```python
from build123d import *

# Parameters (mm, degrees)
F0_R          = 1.75
F1_DEPTH      = 15.875
F3_DEPTH      = 31.75
F4_R          = 3
F5_W          = 5
F5_H          = 35
F6_DEPTH      = 10.001
F6_DEPTH_BACK = 7.5573491861
F7_T1_DEPTH   = 8.7055800262
F7_T3_DEPTH   = 8.75
F7_T5_DEPTH   = 8.75
F7_T7_DEPTH   = 8.7055800262
F8_DEPTH      = 0.2
F9_DEPTH      = 0.2


# Not quite as in the source:
# - a fillet or chamfer that OpenCascade refuses, or shapes differently, is made with other operations: its cross-section is extruded or revolved along the edge and cut away or added


with BuildPart() as f1:
    # F0 (on Right) → F1 (new body, symmetric)
    with BuildSketch(Plane.YZ):
        with BuildLine():
            Line((-5.2303039929, -1.5), (-4.7696960071, -1.5))
            ThreePointArc((-4.7696960071, -1.5), (5, 0), (-4.7696960071, 1.5))
            Line((-4.7696960071, 1.5), (-35, 1.5))
            Line((-35, 1.5), (-42.5, -6))
            Line((-42.5, -6), (-77.5, -6))
            Line((-77.5, -6), (-90.4705627485, 6.9705627485))
            ThreePointArc((-90.4705627485, 6.9705627485), (-93.2989898732, 6.9705627485), (-93.2989898732, 4.1421356237))
            Line((-93.2989898732, 4.1421356237), (-79.1568542495, -10))
            Line((-79.1568542495, -10), (-40.8431457505, -10))
            Line((-40.8431457505, -10), (-32.3431457505, -1.5))
            Line((-32.3431457505, -1.5), (-14.7696960071, -1.5))
            ThreePointArc((-14.7696960071, -1.5), (-10, -5), (-5.2303039929, -1.5))
        make_face()
        Circle(F0_R, mode=Mode.SUBTRACT)
    extrude(amount=F1_DEPTH, both=True)

    # F2 (on face) → F3 (join, through all)
    with BuildSketch(Plane.YZ.offset(15.875)):
        with BuildLine():
            ThreePointArc((-5.2303039929, -1.5), (-7.0419601085, -4.0311288741), (-10, -5))
            Line((-10, -5), (0, -5))
            ThreePointArc((0, -5), (-2.9580398915, -4.0311288741), (-4.7696960071, -1.5))
            Line((-4.7696960071, -1.5), (-5.2303039929, -1.5))
        make_face()
    extrude(amount=-F3_DEPTH)

    # F4
    f4_edges = [f1.edges().sort_by_distance(p)[0] for p in [
        (0, -4.769696, 1.5),
        (0, -14.769696, -1.5),
        (0, -77.5, -6),
        (0, -79.156854, -10),
        (0, -40.843146, -10),
        (0, -32.343146, -1.5),
        (0, -42.5, -6),
        (0, -35, 1.5),
    ]]
    fillet(f4_edges, radius=F4_R)

    # F5 (on Top) → F6 (cut, two sides)
    with BuildSketch(Plane.XY) as f6_sk:
        with Locations((-13.375, -12.5)):
            Rectangle(F5_W, F5_H)
        with Locations((13.375, -12.5)):
            Rectangle(F5_W, F5_H)
    extrude(amount=-F6_DEPTH, mode=Mode.SUBTRACT)
    extrude(f6_sk.sketch, amount=F6_DEPTH_BACK, mode=Mode.SUBTRACT)

    # F7: fillet of radius 1.5 on 4 edges, made by hand

    # F7_s2 → F7_t1 (cut)
    with BuildSketch(Plane.YZ.offset(10.875)):
        with BuildLine():
            ThreePointArc((-31.3668350211, -1.5118453264), (-30.3932598615, -1.0302531824), (-30, -0.0177679895))
            Line((-30, -0.0177679895), (-29.85, -0.0177679895))
            Line((-29.85, -0.0177679895), (-29.85, -1.5))
            Line((-29.85, -1.5), (-30, -1.65))
            ThreePointArc((-30, -1.65), (-31.1005050634, -1.65), (-31.3535185232, -1.66125306))
            Line((-31.3535185232, -1.66125306), (-31.3668350211, -1.5118453264))
        make_face()
    extrude(amount=F7_T1_DEPTH, mode=Mode.SUBTRACT)

    # F7_s4 → F7_t3 (cut)
    with BuildSketch(Plane.YZ.offset(10.875)):
        with BuildLine():
            ThreePointArc((-30, 0), (-30.4393398282, 1.0606601718), (-31.5, 1.5))
            Line((-31.5, 1.5), (-30, 1.5))
            Line((-30, 1.5), (-30, 0))
        make_face()
    extrude(amount=F7_T3_DEPTH, mode=Mode.SUBTRACT)

    # F7_s6 → F7_t5 (cut)
    with BuildSketch(Plane.YZ.offset(-19.625)):
        with BuildLine():
            ThreePointArc((-30, 0), (-30.4393398282, 1.0606601718), (-31.5, 1.5))
            Line((-31.5, 1.5), (-30, 1.5))
            Line((-30, 1.5), (-30, 0))
        make_face()
    extrude(amount=F7_T5_DEPTH, mode=Mode.SUBTRACT)

    # F7_s8 → F7_t7 (cut)
    with BuildSketch(Plane.YZ.offset(-19.5805800262)):
        with BuildLine():
            ThreePointArc((-31.3668350211, -1.5118453264), (-30.3932598615, -1.0302531824), (-30, -0.0177679895))
            Line((-30, -0.0177679895), (-29.85, -0.0177679895))
            Line((-29.85, -0.0177679895), (-29.85, -1.5))
            Line((-29.85, -1.5), (-30, -1.65))
            ThreePointArc((-30, -1.65), (-31.1005050634, -1.65), (-31.3535185232, -1.66125306))
            Line((-31.3535185232, -1.66125306), (-31.3668350211, -1.5118453264))
        make_face()
    extrude(amount=F7_T7_DEPTH, mode=Mode.SUBTRACT)

    # F8 (cut): a face of the model
    f8_faces = [f1.faces().sort_by_distance(p)[0] for p in [
        (10.875, -9.1101781633, -0.6280033564),
    ]]
    extrude(f8_faces, amount=-F8_DEPTH, mode=Mode.SUBTRACT)

    # F9 (cut): a face of the model
    f9_faces = [f1.faces().sort_by_distance(p)[0] for p in [
        (-10.875, -9.1101781633, -0.6280033564),
    ]]
    extrude(f9_faces, amount=-F9_DEPTH, mode=Mode.SUBTRACT)


solid = f1.part
```
The listing builds one solid part. Answer for the finished solid, in the listing's coordinates (mm). A direction names the side the tool comes from. Coordinates: 2 decimals unless noted, no trailing zeros. Loops run counter-clockwise (first coordinate to the right, second up) from the corner with the lowest first, then second, coordinate; pieces in that order, holes last. Notation, with made-up numbers: M 13,1 L 47,1 A25 cw 47,13 Z; hole C 75.5,26 d10. An arc over 180 degrees is marked long. Answer as CSV lines item,"result". Start each with the question number.
(1) The part is cut by section C-C (z = -7.5). Give the vertices of the cut face in (x, y) (3 decimals), and give its area (3 significant figures).
(2) The part is cut by section A-A (x = 4). Give the vertices of the cut face in (y, z).
(3) Given pin 1 (5.5 mm diameter, centred on y = 0, z = 0, fed in from -X) (3 decimals); pin 2 (4 mm diameter, centred on x = 3.5, z = -6, fed in from +Y); pin 3 (5 mm diameter, centred on x = 4, y = -7, fed in from -Z); pin 4 (5 mm diameter, centred on y = -64.5, z = -4.5, fed in from +X) (3 decimals), each flat-ended and moving along its own axis, determine where each tip first touches the part or whether it passes through.
(4) For faces 1 (the flat face through (15.875, -62.1, -6.4)), 2 (the flat face through (0.2, -84.3, 0.8)), 3 (the cylindrical face through (-0.15, -15.19, -1.86)), determine the directions among +Z, -Z, +X, -X, +Y, -Y from which every point of the face is accessible in a straight line to the end or side of a thin tool.
(5) Find the intervals of material crossed by L1, parallel to Z at x = -4, y = 0; L2, parallel to Y at x = -4.5, z = 0; L3, parallel to Y at x = -7, z = 2.5, in increasing order. Write a range as [from, to].
(6) The mould has two halves that part along Y. Classify faces 4 (the cylindrical face through (0.22, -93.27, 7)), 5 (the flat face through (0, -5, -5)), 6 (the cylindrical face through (0.15, -5.19, 1.86)): pulls with the +Y half, pulls with the -Y half, needs draft (parallel to the pull), parting line crosses it, or undercut.
(7) The part is cut by section B-B (y = -8.5). Give the vertices of the cut face in (x, z) (3 decimals), and give its area (3 significant figures).
Determined:
1,outline,"M -15.875,-81.657 L 15.875,-81.657 L 15.875,-38.343 L -15.875,-38.343 Z"
1,area,"1,380 mm2"
2,outline,"M -93.3,4.14 L -80.04,-9.12 A3 ccw -77.91,-10 L -42.09,-10 A3 ccw -39.96,-9.12 L -33.22,-2.38 A3 cw -31.1,-1.5 L -16.61,-1.5 A3 cw -14.13,-2.81 A5 ccw -10,-5 L 0,-5 A5 ccw long -4.13,2.81 A3 cw -6.61,1.5 L -33.76,1.5 A3 ccw -35.88,0.62 L -41.62,-5.12 A3 cw -43.74,-6 L -76.26,-6 A3 cw -78.38,-5.12 L -90.47,6.97 A2 ccw Z; hole C 0,0 d3.5"
3,pin 1,"x = -10.675"
3,pin 2,"y = 3"
3,pin 3,"z = -5"
3,pin 4,"x = 15.875"
4,face 1,"+Z, -Z, +X, +Y, -Y"
4,face 2,"+Z, +X, -X"
4,face 3,"-Z, +X, -X"
5,L1,"[-5, -1.75], [1.75, 5]"
5,L2,"[-89.16, -83.5], [-36.5, -1.75], [1.75, 5]"
5,L3,"[-91.66, -86], [-4.38, 4.33]"
6,face 4,"parting line crosses it"
6,face 5,"needs draft"
6,face 6,"undercut"
7,outline,"M -10.675,-5 L 10.675,-5 L 10.675,1.5 L -10.675,1.5 Z"
7,area,"139 mm2"
